Design review of the part shown in the three views and the two pictorial views. Dimensions are in mm from the part's minimum x, y and z. Coordinates: 2 decimals unless noted, no trailing zeros. Loops run counter-clockwise (first coordinate to the right, second up) from the corner with the lowest first, then second, coordinate; pieces in that order, holes last. Notation, with made-up numbers: (50, 72.5) -> (64, 72.5) arc R4 ccw to (64, 79.5) -> close; hole circle Ø2 at (85.5, 40.5). An arc over 180 degrees is marked (long way). One line per item, written item: value. Start each with the question number.
1. Add section A-A on z = 24.5. Write out the cut boundary in (x, y).
2. For probe 1 along X at (y, z) = (3, 44) (1 decimal); probe 2 along Z at (x, y) = (4.25, 3.5); probe 3 along X at (y, z) = (3.3, 6) (1 decimal), list the stretches that pass through material, from the lowest coordinate up.
3. Add section C-C on x = 0.5. Write out the cut boundary in (y, z), plus the area to 3 significant figures.
4. Insertion check: pin 1 (1.5 mm diameter, centred on y = 4, z = 16, fed in from +X); pin 2 (1.5 mm diameter, centred on y = 4.5, z = 45, fed in from +X) (1 decimal). Each pin has a flat end and moves straight along its axis. Give the tip position at first contact, or say it passes through.
5. Add section B-B on x = 6.25. Write out the cut boundary in (y, z) (1 decimal).
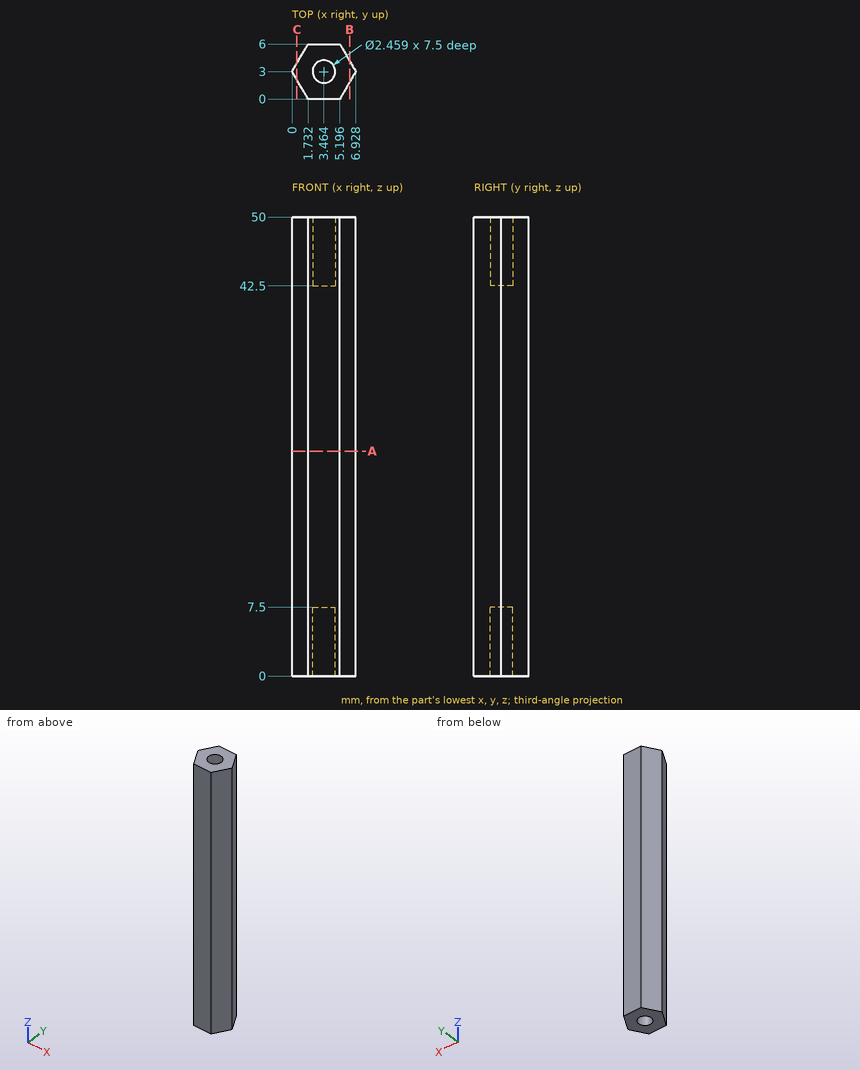
Worked answers:
1. outline: (0, 3) -> (1.73, 0) -> (5.2, 0) -> (6.93, 3) -> (5.2, 6) -> (1.73, 6) -> close
2. probe 1: x = 0 to 2.2, 4.7 to 6.9
2. probe 2: z = 7.5 to 42.5
2. probe 3: x = 0.2 to 2.3, 4.7 to 6.8
3. outline: (2.13, 0) -> (3.87, 0) -> (3.87, 50) -> (2.13, 50) -> close
3. area: 86.6 mm²
4. pin 1: stops at x = 6.78
4. pin 2: stops at x = 6.5
5. outline: (1.8, 0) -> (4.2, 0) -> (4.2, 50) -> (1.8, 50) -> close
